```python
from build123d import *

# Parameters (mm, degrees)
SWEEP2_PROFILE_R        = 5
CUT_EXTRUDE1_DEPTH      = 77.321687612
CUT_EXTRUDE1_DEPTH_BACK = 77.321687612
SKETCH4_W               = 8
SKETCH4_H               = 4


with BuildPart() as part:
    # Sweep2: sweep along a path in Sketch2
    with BuildLine(Plane(origin=(0, 0, 0), x_dir=(1, 0, 0), z_dir=(0, 1, 0))) as sweep2_path:
        Line((0, 70), (0, -10))
        Line((0, -10), (30, -10))
    # Sweep2 profile (on start of the path) → Sweep2 (sweep)
    with BuildSketch(Plane.XY.offset(-70)):
        Circle(SWEEP2_PROFILE_R)
    sweep(path=sweep2_path.line, transition=Transition.RIGHT)

    # Sketch4 → Cut-Extrude1 (cut, two sides: drawn at the far end of the back side and taken through both)
    with BuildSketch(Plane(origin=(0, 0, 0), x_dir=(0, 0, -1), z_dir=(1, 0, 0)).offset(-CUT_EXTRUDE1_DEPTH_BACK)):
        with Locations((35, 0)):
            Rectangle(SKETCH4_W, SKETCH4_H)
    extrude(amount=CUT_EXTRUDE1_DEPTH + CUT_EXTRUDE1_DEPTH_BACK, mode=Mode.SUBTRACT)


solid = part.part
```
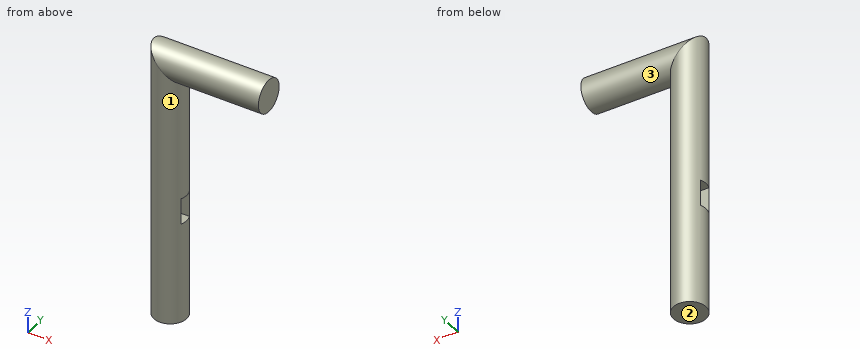
Could you check a few things on this model? Use its own coordinates, in mm. Face numbers are marked on the shaded views. A direction names the side the tool comes from. Round coordinates to 2 decimals unless told otherwise and drop trailing zeros. Loops run counter-clockwise (first coordinate to the right, second up) from the corner with the lowest first, then second, coordinate; pieces in that order, holes last. Notation, with made-up numbers: (71, 56.25) - (80, 56.25) arc R11 ccw to (80, 73.25) - close; hole circle Ø5 at (-15, -39). An arc over 180 degrees is marked (long way). Use CSV: the item, a comma, the result in double quotes.
Item 1: If we section it at C-C on z = -58: List the corners of the cut face in (x, y) for me, then the cut area to 3 significant figures.
Here are the results:
outline,"circle Ø10 at (0, 0)"
area,"78.5 mm²"
Item 2: For the marked faces 1, 2 and 3, which set-ups out of +Z, -Z, +X, -X, +Y, -Y let a thin tool reach every point of the face, with its end or its side?
Here are the results:
face 1,"-Z"
face 2,"-Z, +X, -X, +Y, -Y"
face 3,"+X"
Item 3: If we section it at B-B on y = -1: List the corners of the cut face in (x, z) for me, then the cut area to 3 significant figures.
Here are the results:
outline,"(-4.9, -70) - (4.9, -70) - (4.9, -39) - (-4.9, -39) - close; (-4.9, -31) - (4.9, -31) - (4.9, 5.1) - (30, 5.1) - (30, 14.9) - (-4.9, 14.9) - close"
area,"999 mm²"
Item 4: If we section it at D-D on y = 3: List the corners of the cut face in (x, z) for me, then the cut area to 3 significant figures.
Here are the results:
outline,"(-4, -70) - (4, -70) - (4, 6) - (30, 6) - (30, 14) - (-4, 14) - close"
area,"880 mm²"
Item 5: If we section it at A-A on x = 0: List the corners of the cut face in (y, z) for me.
Here are the results:
outline,"(-5, -70) - (5, -70) - (5, 10) arc R5 ccw to (-5, 10) - close; hole (-2, -39) - (2, -39) - (2, -31) - (-2, -31) - close"
Item 6: Will these pins go through, and if not, where does the flat tip stop? pin 1 (1 mm diameter, centred on x = -1.5, z = -33, fed in from -Y); pin 2 (1.5 mm diameter, centred on y = 2, z = -59.5, fed in from -X); pin 3 (1 mm diameter, centred on x = 8.5, y = 3, fed in from -Z).
Here are the results:
pin 1,"stops at y = -4.9"
pin 2,"stops at x = -4.84"
pin 3,"stops at z = 5.67"
Item 7: I need wall thicknesses on L1, parallel to X at y = -2, z = -63; L2, parallel to X at y = -0.25, z = 1.5; L3, parallel to Y at x = 4.5, z = -22.5. Which ranges of each line are inside material? Lowest first, please. Write a range as [from, to].
Here are the results:
L1,"x = [-4.58, 4.58]"
L2,"x = [-4.99, 4.99]"
L3,"y = [-2.18, 2.18]"
